For this review, use the dimensioned drawing (mm, ordinates from the lowest corner) and the shaded views. Coordinates: 2 decimals unless noted, no trailing zeros. Loops run counter-clockwise (first coordinate to the right, second up) from the corner with the lowest first, then second, coordinate; pieces in that order, holes last. Notation, with made-up numbers: M 19,70.25 L 25,70.25 A29 cw 25,101.25 Z; hole C 7.5,85 d9. An arc over 180 degrees is marked long. One line per item, written item: value.
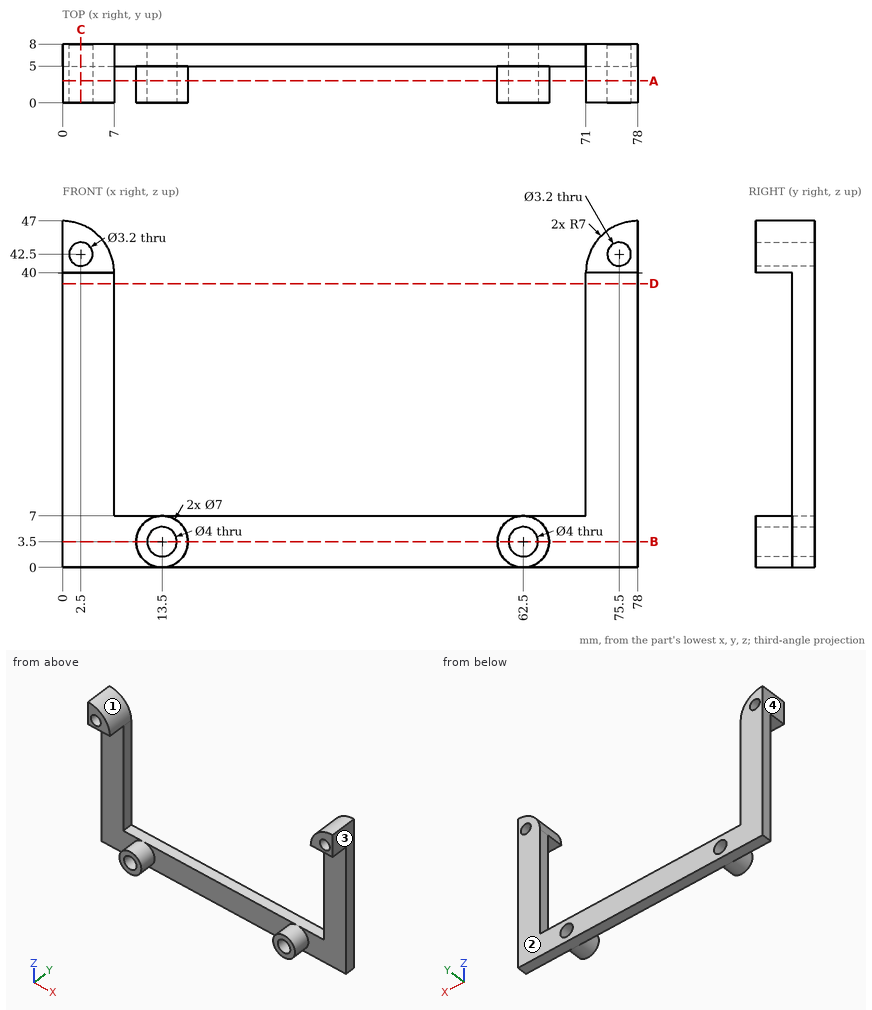
(1) Add section A-A on y = 3. State the section outline as (x, z) points, then the cut area to 3 significant figures.
Checks:
outline: M 0,40 L 7,40 A7 ccw 0,47 Z; C 13.5,3.5 d7; C 62.5,3.5 d7; M 71,40 L 78,40 L 78,47 A7 ccw Z; hole C 2.5,42.5 d3.2; hole C 13.5,3.5 d4; hole C 62.5,3.5 d4; hole C 75.5,42.5 d3.2
area: 113 mm^2
(2) Add section B-B on z = 3.5. State the section outline as (x, y) points, then the cut area to 3 significant figures.
Checks:
outline: M 0,5 L 10,5 L 10,0 L 11.5,0 L 11.5,8 L 0,8 Z; M 15.5,0 L 17,0 L 17,5 L 59,5 L 59,0 L 60.5,0 L 60.5,8 L 15.5,8 Z; M 64.5,0 L 66,0 L 66,5 L 78,5 L 78,8 L 64.5,8 Z
area: 240 mm^2
(3) Add section D-D on z = 38.5. State the section outline as (x, y) points.
Checks:
outline: M 0,5 L 7,5 L 7,8 L 0,8 Z; M 71,5 L 78,5 L 78,8 L 71,8 Z
(4) Draft analysis for pull direction X (two halves, no side actions). For the marked faces 1, 2, 3 and 4, state which applies: pulls with the +X half, pulls with the -X half, needs draft (parallel to the pull), parting line crosses it, or undercut.
Checks:
face 1: undercut
face 2: needs draft
face 3: pulls with the +X half
face 4: pulls with the -X half
(5) Insertion check: pin 1 Ø3 at (x, z) = (75.5, 42.5) entering from +Y; pin 2 Ø17 at (x, z) = (68, 15.5) entering from -Y; pin 3 Ø0.9 at (x, y) = (43, 7) entering from +Z. Each pin has a flat end and moves straight along its axis. Give the tip position at first contact, or say it passes through.
Checks:
pin 1: through
pin 2: y = 5
pin 3: z = 7
(6) Add section C-C on x = 2.5. State the section outline as (y, z) points, then the cut area to 3 significant figures.
Checks:
outline: M 0,40 L 5,40 L 5,0 L 8,0 L 8,40.9 L 0,40.9 Z; M 0,44.1 L 8,44.1 L 8,46.54 L 0,46.54 Z
area: 147 mm^2
(7) To check wall thickness, follow L1, parallel to Z at x = 29.5, y = 7.5; L2, parallel to Y at x = 22, z = 4; L3, parallel to X at y = 7.75, z = 31.5. State the ranges of each line that lie inside material, in increasing order. Write a range as [from, to].
Checks:
L1: [0, 7]
L2: [5, 8]
L3: [0, 7], [71, 78]
